Check sheet for the modelled part. Datum: model origin and axes. Units: mm. A direction names the side the tool comes from. Round coordinates to 2 decimals unless told otherwise and drop trailing zeros. Write each loop counter-clockwise with the first axis right and the second up, starting at its lowest first coordinate (ties: lowest second). Pieces come first, ordered by that corner, then holes.
from build123d import *

# Parameters (mm, degrees)
F0_W      = 12
F0_H      = 238
F0_H_2    = 12
F0_W_2    = 166
F0_H_3    = 272
F1_DEPTH  = 224
F2_R      = 24
F3_R      = 36
F5_DEPTH  = 12
F7_DEPTH  = 12
F8_R      = 63
F9_DEPTH  = 190
F10_R     = 11
F11_DEPTH = 25
F12_R     = 5
F13_DEPTH = 25


with BuildPart() as f1:
    # F0 (on Front) → F1 (new body)
    with BuildSketch(Plane.XZ):
        with Locations((-29.668833, 69.198049)):
            Rectangle(F0_W, F0_H)
        with Locations((-29.668833, -55.801951)):
            Rectangle(F0_W, F0_H_2)
        with Locations((59.331167, -55.801951)):
            Rectangle(F0_W_2, F0_H_2)
        with Locations((148.331167, 86.198049)):
            Rectangle(F0_W, F0_H_3)
        with Locations((148.331167, -55.801951)):
            Rectangle(F0_W, F0_H_2)
    extrude(amount=F1_DEPTH)

    # F2
    f2_edges = [f1.edges().sort_by_distance(p)[0] for p in [
        (-23.668833, -112, -49.801951),
        (142.331167, -112, -49.801951),
    ]]
    fillet(f2_edges, radius=F2_R)

    # F3
    f3_edges = [f1.edges().sort_by_distance(p)[0] for p in [
        (154.331167, -112, -61.801951),
        (-35.668833, -112, -61.801951),
    ]]
    fillet(f3_edges, radius=F3_R)

    # F4 (on face) → F5 (cut)
    with BuildSketch(Plane(origin=(-35.668833, 0, 0), x_dir=(0, -1, 0), z_dir=(-1, 0, 0))):
        Polygon((0, 114.333307), (40, 188.198049), (0, 188.198049), align=None)
        Polygon((224, 188.198049), (184, 188.198049), (224, 114.333307), align=None)
    extrude(amount=-F5_DEPTH, mode=Mode.SUBTRACT)

    # F6 (on face) → F7 (cut)
    with BuildSketch(Plane.YZ.offset(154.331167)):
        Polygon((-224, 222.198049), (-224, 157.576071), (-184, 222.198049), align=None)
        Polygon((0, 222.198049), (-40, 222.198049), (0, 157.576071), align=None)
    extrude(amount=-F7_DEPTH, mode=Mode.SUBTRACT)

    # F8 (on face) → F9 (cut)
    with BuildSketch(Plane(origin=(-35.668833, 0, 0), x_dir=(0, -1, 0), z_dir=(-1, 0, 0))):
        with Locations((112, 113.482498)):
            Circle(F8_R)
    extrude(amount=-F9_DEPTH, mode=Mode.SUBTRACT)

    # F10 (on face) → F11 (cut)
    with BuildSketch(Plane.YZ.offset(154.331167)):
        with Locations((-166, 200.198049)):
            Circle(F10_R)
        with Locations((-58, 200.198049)):
            Circle(F10_R)
        with Locations((-34, 30.198049)):
            Circle(F10_R)
        with Locations((-190, 30.198049)):
            Circle(F10_R)
    extrude(amount=-F11_DEPTH, mode=Mode.SUBTRACT)

    # F12 (on face) → F13 (cut)
    with BuildSketch(Plane.XY.offset(-49.801951)):
        with Locations((69.331167, -204)):
            Circle(F12_R)
        with Locations((69.331167, -20)):
            Circle(F12_R)
    extrude(amount=-F13_DEPTH, mode=Mode.SUBTRACT)


solid = f1.part
1. Sectioned sample at A-A, the plane z = 63. Enter the section's corners in (x, y).
2. Set-up check for faces 5 (the flat face through (-30, -111, 188.198)), 6 (the flat face through (-23.669, -85.5, 55.9)), 7 (the flat face through (-29.75, -19.72, 150.75)), 8 (the flat face through (-29.75, -203.72, 151.78)): record each of +Z, -Z, +X, -X, +Y, -Y from which the full face is reachable in a straight line by a thin tool's end or side.
3. Sectioned sample at D-D, the plane y = -190. Enter the section's corners in (x, z).
4. Go/stop test with flat-tipped pins: pin 1 (4 mm diameter, centred on x = 74, y = -184, fed in from +Z); pin 2 (20 mm diameter, centred on y = -190, z = 30.2, fed in from +X); pin 3 (5 mm diameter, centred on x = 130, y = -172.5, fed in from +Z). Record where each tip stops, or that it passes through.
5. Release check for a two-part mould opening along Y. For faces 1 (the cylindrical face through (148.42, -200.99, 30.68)), 2 (the flat face through (143, 0, 24)), 3 (the cylindrical face through (-29.753, -103.799, 175.946)), 4 (the flat face through (143, -224, 24)) record: released by +Y, released by -Y, zero draft, split by the parting line, or undercut.
6. Scan lines: line 1 along X through (y, z) = (-30.5, 114); line 2 along Z through (x, y) = (145, -166); line 3 along X through (y, z) = (-213, -47). Record each from-to range of solid material in increasing order.
7. Sectioned sample at B-B, the plane y = -142. Enter the section's corners in (x, z).
8. Sectioned sample at C-C, the plane y = -58. Enter the section's corners in (x, z), plus the area to 3 significant figures.
Computed values:
1. outline: (-35.67, -224) - (-23.67, -224) - (-23.67, -149.69) - (-35.67, -149.69) - close; (-35.67, -74.31) - (-23.67, -74.31) - (-23.67, 0) - (-35.67, 0) - close; (142.33, -224) - (154.33, -224) - (154.33, -149.69) - (142.33, -149.69) - close; (142.33, -74.31) - (154.33, -74.31) - (154.33, 0) - (142.33, 0) - close
2. face 5: +Z, -X, +Y, -Y
2. face 6: +Z, +Y, -Y
2. face 7: +Z, -X, +Y
2. face 8: +Z, -X, -Y
3. outline: (-35.67, -25.8) arc R36 ccw to (0.33, -61.8) - (118.33, -61.8) arc R36 ccw to (154.33, -25.8) - (154.33, 19.2) - (142.33, 19.2) - (142.33, -25.8) arc R24 cw to (118.33, -49.8) - (0.33, -49.8) arc R24 cw to (-23.67, -25.8) - (-23.67, 177.12) - (-35.67, 177.12) - close; (142.33, 41.2) - (154.33, 41.2) - (154.33, 212.5) - (142.33, 212.5) - close
4. pin 1: stops at z = -49.8
4. pin 2: stops at x = -23.67
4. pin 3: stops at z = -45.17
5. face 1: undercut
5. face 2: released by +Y
5. face 3: undercut
5. face 4: released by -Y
6. line 1: x = -35.67 to -23.67, 142.33 to 154.33
6. line 2: z = -49.98 to 81.03, 145.93 to 189.2, 211.2 to 222.2
6. line 3: x = -28.77 to -10.92, 129.58 to 147.43
7. outline: (-35.67, -25.8) arc R36 ccw to (0.33, -61.8) - (118.33, -61.8) arc R36 ccw to (154.33, -25.8) - (154.33, 58.08) - (142.33, 58.08) - (142.33, -25.8) arc R24 cw to (118.33, -49.8) - (0.33, -49.8) arc R24 cw to (-23.67, -25.8) - (-23.67, 58.08) - (-35.67, 58.08) - close; (-35.67, 168.88) - (-23.67, 168.88) - (-23.67, 188.2) - (-35.67, 188.2) - close; (142.33, 168.88) - (154.33, 168.88) - (154.33, 222.2) - (142.33, 222.2) - close
8. outline: (-35.67, -25.8) arc R36 ccw to (0.33, -61.8) - (118.33, -61.8) arc R36 ccw to (154.33, -25.8) - (154.33, 81.03) - (142.33, 81.03) - (142.33, -25.8) arc R24 cw to (118.33, -49.8) - (0.33, -49.8) arc R24 cw to (-23.67, -25.8) - (-23.67, 81.03) - (-35.67, 81.03) - close; (-35.67, 145.93) - (-23.67, 145.93) - (-23.67, 188.2) - (-35.67, 188.2) - close; (142.33, 145.93) - (154.33, 145.93) - (154.33, 189.2) - (142.33, 189.2) - close; (142.33, 211.2) - (154.33, 211.2) - (154.33, 222.2) - (142.33, 222.2) - close
8. area: 6,270 mm2
